```python
from build123d import *

# Parameters (mm, degrees)
SKETCH1_R           = 20
BOSS_EXTRUDE1_DEPTH = 457
SKETCH2_R           = 10
CUT_EXTRUDE1_DEPTH  = 526
SKETCH6_R           = 20
BOSS_EXTRUDE4_DEPTH = 82
SKETCH7_W           = 75
SKETCH7_H           = 40
BOSS_EXTRUDE5_DEPTH = 20


with BuildPart() as part:
    # Sketch1 → Boss-Extrude1 (new body)
    with BuildSketch(Plane(origin=(0, 0, 0), x_dir=(1, 0, 0), z_dir=(0, 1, 0))):
        Circle(SKETCH1_R)
    extrude(amount=BOSS_EXTRUDE1_DEPTH)

    # Sketch2 → Cut-Extrude1 (cut)
    with BuildSketch(Plane(origin=(0, 457, 0), x_dir=(1, 0, 0), z_dir=(0, 1, 0))):
        Circle(SKETCH2_R)
    extrude(amount=-CUT_EXTRUDE1_DEPTH, mode=Mode.SUBTRACT)

    # Sketch6 → Boss-Extrude4 (add)
    with BuildSketch(Plane.XZ):
        with Locations((35, 0)):
            Circle(SKETCH6_R)
    extrude(amount=-BOSS_EXTRUDE4_DEPTH)

    # Sketch7 → Boss-Extrude5 (add)
    with BuildSketch(Plane.XZ):
        with Locations((17.5, 0)):
            Rectangle(SKETCH7_W, SKETCH7_H)
    extrude(amount=-BOSS_EXTRUDE5_DEPTH)


solid = part.part
```
Here's how the part is built. I have some questions about the finished solid (model axes, mm). A direction names the side the tool comes from. Coordinates: 2 decimals unless noted, no trailing zeros. Order: outer loops, then holes, each group sorted by start corner. A loop starts at its lowest first (then second) coordinate and runs counter-clockwise, first axis right, second up.
Item 1: If we section it at C-C, the plane x = -5: List the corners of the cut face in (y, z) for me.
Response values:
outline: (0, -20) - (20, -20) - (20, -19.36) - (457, -19.36) - (457, -8.66) - (20, -8.66) - (20, 8.66) - (457, 8.66) - (457, 19.36) - (20, 19.36) - (20, 20) - (0, 20) - close
Item 2: Thinking about a two-plate mould opening in X: for faces 1 (the face through (17, 0, 0)), 2 (the face through (17, 20, 17)), 3 (the face through (-2.17, 241.56, 9.76)), 4 (the face through (-20, 10, 0)), which applies, pulls with the +X half, pulls with the -X half, needs draft (parallel to the pull), parting line crosses it, or undercut?
Response values:
face 1: needs draft
face 2: undercut
face 3: undercut
face 4: pulls with the -X half
Item 3: I need wall thicknesses on probe 1 along X at (y, z) = (248.5, 0); probe 2 along X at (y, z) = (423, 1). Which ranges of each line are inside material? Lowest first, please.
Response values:
probe 1: x = -20 to -10, 10 to 20
probe 2: x = -19.97 to -9.95, 9.95 to 19.97
Item 4: Which directions (+Z, -Z, +X, -X, +Y, -Y) give clear straight access to the entire face, cutting with the end or side of a thin tool? Please do faces 5 (the face through (17, 20, -17)), 6 (the face through (51, 20, -16)), 7 (the face through (-16, 20, -15)).
Response values:
face 5: -Z, +Y
face 6: -Z, +X, +Y
face 7: -Z, -X, +Y
Item 5: If we section it at B-B, the plane x = 40.5: List the corners of the cut face in (y, z) for me.
Response values:
outline: (0, -20) - (20, -20) - (20, -19.23) - (82, -19.23) - (82, 19.23) - (20, 19.23) - (20, 20) - (0, 20) - close
Item 6: If we section it at A-A, the plane y = 223.5: List the corners of the cut face in (x, z) for me.
Response values:
outline: circle Ø40 at (0, 0); hole circle Ø20 at (0, 0)
Item 7: I'm going to push flat-ended pins straight in: pin 1 Ø3 at (y, z) = (252.5, 7) entering from -X; pin 2 Ø3 at (x, y) = (-4, 411.5) entering from -Z; pin 3 Ø10 at (x, z) = (42.5, 11.5) entering from +Y. Where does each tip first touch, or does it pass through?
Response values:
pin 1: stops at x = -19.23
pin 2: stops at z = -19.84
pin 3: stops at y = 82
